Input: part model. Units: mm. Frame: model coordinates. A direction names the side the tool comes from. Give positions to 0.01 mm unless a question says otherwise; leave off trailing zeros. Loops run counter-clockwise (first coordinate to the right, second up) from the corner with the lowest first, then second, coordinate; pieces in that order, holes last. Notation, with made-up numbers: (88, -25) - (103, -25) arc R24 ccw to (103, 7) - close; hole circle Ø5 at (38.5, 36). An arc over 180 degrees is marked (long way). Answer as a JSON object with one key per item and string values.
from build123d import *

# Parameters (mm, degrees)
ESQUISSE1_R                  = 2
BOSS_EXTRU_1_DEPTH           = 4
BOSS_EXTRU_2_DEPTH           = 30
BOSS_EXTRU_2_DEPTH_BACK      = 30
ENL_V_MAT_EXTRU_1_REACH      = 23.158
ESQUISSE3_R                  = 1.75
CONG_1_R                     = 6
CONG_2_R                     = 5
ESQUISSE4_W                  = 40
ESQUISSE4_H                  = 20
ENL_V_MAT_EXTRU_2_DEPTH      = 15
ENL_V_MAT_EXTRU_2_DEPTH_BACK = 22
ESQUISSE5_W                  = 40
ESQUISSE5_H                  = 7.135689783
BOSS_EXTRU_3_DEPTH           = 4
CONG_4_R                     = 6
CONG_5_R                     = 4


with BuildPart() as part:
    # Esquisse1 → Boss.-Extru.1 (new body)
    with BuildSketch(Plane(origin=(0, 0, 0), x_dir=(1, 0, 0), z_dir=(0, 1, 0))):
        with BuildLine():
            Line((-45, 15), (45, 15))
            ThreePointArc((45, 15), (52.071067812, 12.071067812), (55, 5))
            Line((55, 5), (55, -5))
            ThreePointArc((55, -5), (52.071067812, -12.071067812), (45, -15))
            Line((45, -15), (-45, -15))
            ThreePointArc((-45, -15), (-52.071067812, -12.071067812), (-55, -5))
            Line((-55, -5), (-55, 5))
            ThreePointArc((-55, 5), (-52.071067812, 12.071067812), (-45, 15))
        make_face()
        with Locations((-45, 0)):
            Circle(ESQUISSE1_R, mode=Mode.SUBTRACT)
        with Locations((45, 0)):
            Circle(ESQUISSE1_R, mode=Mode.SUBTRACT)
    extrude(amount=BOSS_EXTRU_1_DEPTH)

    # Esquisse2 → Boss.-Extru.2 (add, two sides)
    with BuildSketch(Plane(origin=(0, 0, 0), x_dir=(0, 0, -1), z_dir=(1, 0, 0))) as boss_extru_2_sk:
        Polygon((-6, 4), (1.488067553, 25.746927239), (5.270141855, 24.444654621), (-1.769517275, 4), align=None)
    extrude(amount=BOSS_EXTRU_2_DEPTH)
    extrude(boss_extru_2_sk.sketch, amount=-BOSS_EXTRU_2_DEPTH_BACK)

    # Esquisse3 → Enlèv. mat.-Extru.1 (cut, up to next)
    with BuildSketch(Plane(origin=(0, 2.270962919, 6.595355211), x_dir=(1, 0, 0), z_dir=(0, 0.325568154, 0.945518576)), mode=Mode.PRIVATE) as enl_v_mat_extru_1_sk1:
        with Locations((22.5, 18.828665376)):
            Circle(ESQUISSE3_R)
    enl_v_mat_extru_1_tool1 = extrude(enl_v_mat_extru_1_sk1.sketch, amount=-ENL_V_MAT_EXTRU_1_REACH, mode=Mode.PRIVATE) & part.part
    add(enl_v_mat_extru_1_tool1.solids().sort_by_distance((22.5, 20.073816, 0.465341))[0], mode=Mode.SUBTRACT)
    # Esquisse3 → Enlèv. mat.-Extru.1 (cut, up to next)
    with BuildSketch(Plane(origin=(0, 2.270962919, 6.595355211), x_dir=(1, 0, 0), z_dir=(0, 0.325568154, 0.945518576)), mode=Mode.PRIVATE) as enl_v_mat_extru_1_sk2:
        with Locations((-22.5, 18.828665376)):
            Circle(ESQUISSE3_R)
    enl_v_mat_extru_1_tool2 = extrude(enl_v_mat_extru_1_sk2.sketch, amount=-ENL_V_MAT_EXTRU_1_REACH, mode=Mode.PRIVATE) & part.part
    add(enl_v_mat_extru_1_tool2.solids().sort_by_distance((-22.5, 20.073816, 0.465341))[0], mode=Mode.SUBTRACT)

    # Congé1
    cong_1_edges = [part.edges().sort_by_distance(p)[0] for p in [
        (-30, 4, 3.884758638),
        (-30, 25.09579093, -3.379104704),
        (30, 4, 3.884758638),
        (30, 25.09579093, -3.379104704),
    ]]
    fillet(cong_1_edges, radius=CONG_1_R)

    # Congé2
    cong_2_edges = [part.edges().sort_by_distance(p)[0] for p in [
        (0, 4, 1.769517275),
    ]]
    fillet(cong_2_edges, radius=CONG_2_R)

    # Esquisse4 → Enlèv. mat.-Extru.2 (cut, two sides)
    with BuildSketch(Plane(origin=(0, 4, 0), x_dir=(1, 0, 0), z_dir=(0, 1, 0))) as enl_v_mat_extru_2_sk:
        Rectangle(ESQUISSE4_W, ESQUISSE4_H)
    extrude(amount=ENL_V_MAT_EXTRU_2_DEPTH, mode=Mode.SUBTRACT)
    extrude(enl_v_mat_extru_2_sk.sketch, amount=-ENL_V_MAT_EXTRU_2_DEPTH_BACK, mode=Mode.SUBTRACT)

    # Esquisse5 → Boss.-Extru.3 (add)
    with BuildSketch(Plane(origin=(0, 2.270962919, 6.595355211), x_dir=(1, 0, 0), z_dir=(0, 0.325568154, 0.945518576))):
        with Locations((0, 21.260820485)):
            Rectangle(ESQUISSE5_W, ESQUISSE5_H)
    extrude(amount=-BOSS_EXTRU_3_DEPTH)

    # Congé4
    cong_4_edges = [part.edges().sort_by_distance(p)[0] for p in [
        (-20, 18.348863691, -1.055951351),
        (20, 18.348863691, -1.055951351),
    ]]
    fillet(cong_4_edges, radius=CONG_4_R)

    # Congé5
    cong_5_edges = [part.edges().sort_by_distance(p)[0] for p in [
        (-20, 2, 10),
        (20, 2, -10),
        (-20, 2, -10),
        (20, 2, 10),
    ]]
    fillet(cong_5_edges, radius=CONG_5_R)


solid = part.part
Item 1: Cut plane A-A (z = -9). Return loops of the section in (x, y), then the cut area to 3 significant figures.
Geometry check:
{"outline": "(-54.17, 0) - (-18.65, 0) - (-18.65, 4) - (-54.17, 4) - close; (18.65, 0) - (54.17, 0) - (54.17, 4) - (18.65, 4) - close", "area": "284 mm2"}
Item 2: Material intervals for line 1 (X direction, y = 2.8, z = 0); line 2 (Z direction, x = 45, y = 1); line 3 (Y direction, x = 40, z = 2.5), sorted ascending. Write a range as [from, to].
Geometry check:
{"line 1": "x = [-55, -47], [-43, -20], [20, 43], [47, 55]", "line 2": "z = [-15, -2], [2, 15]", "line 3": "y = [0, 4]"}
Item 3: Cut plane D-D (x = -28.5). Return loops of the section in (y, z), then the cut area to 3 significant figures.
Geometry check:
{"outline": "(0, -15) - (4, -15) - (4, -5.24) arc R5 cw to (10.63, -0.51) - (22.52, -4.61) - (23.83, -0.83) - (4, 6) - (4, 15) - (0, 15) - close", "area": "212 mm2"}
Item 4: Mould query, pull axis Z, two halves, no side actions, for faces 5 (the face through (-52.15, 1.97, -11.99)), 6 (the face through (18.797, 1.972, -8.859)), 7 (the face through (-0.196, 18.358, -1.029)). Classes: released by +Z, released by -Z, zero draft, split by the parting line, or undercut.
Geometry check:
{"face 5": "released by -Z", "face 6": "undercut", "face 7": "released by +Z"}
Item 5: Cut plane B-B (x = 22.5). Return loops of the section in (y, z), then the cut area to 3 significant figures.
Geometry check:
{"outline": "(0, -15) - (4, -15) - (4, -5.24) arc R5 cw to (10.63, -0.51) - (17.12, -2.75) - (18.42, 1.04) - (4, 6) - (4, 15) - (0, 15) - close; (20.43, -3.89) - (24.44, -5.27) - (25.75, -1.49) - (21.73, -0.1) - close", "area": "207 mm2"}
Item 6: Cut plane C-C (x = -39.5). Return loops of the section in (y, z).
Geometry check:
{"outline": "(0, -15) - (4, -15) - (4, 15) - (0, 15) - close"}
Item 7: Access query for faces 1 (the face through (20, 5, 1)), 2 (the face through (30, 15, 0)), 3 (the face through (-30, 15, 0)), 4 (the face through (18.797, 1.972, 8.859)). Directions: +Z, -Z, +X, -X, +Y, -Y. A direction counts if a zero-diameter tool reaches every point of the face in a straight line with its end or side. Return the directions, or none.
Geometry check:
{"face 1": "-Y", "face 2": "+Z, -Z, +X, +Y", "face 3": "+Z, -Z, -X, +Y", "face 4": "+Y, -Y"}
Item 8: Contact query for flat-ended pins moving along their axis: P1, Ø2.5, axis at x = 45, z = 0, coming from the +Y side; P2, Ø2, axis at y = 12.5, z = -1, coming from the -X side; P3, Ø3.5, axis at y = 16.5, z = 0.5, coming from the +X side; P4, Ø9.5, axis at y = 9.5, z = 2.5, coming from the -X side. Output: stop coordinate, or through.
Geometry check:
{"P1": "passes through", "P2": "stops at x = -30", "P3": "stops at x = 30", "P4": "stops at x = -33.1"}
